from build123d import *

# Parameters (mm, degrees)
SKETCH_1_W          = 57
SKETCH_1_H          = 57
EXTRUDE_1_DEPTH     = 112
FILLET_1_R          = 2
CUT_EXTRUDE_2_DEPTH = 107.3
SKETCH_6_R          = 4
EXTRUDE_2_DEPTH     = 20
SKETCH_7_W          = 9.44271558
SKETCH_7_H          = 0.5
CUT_EXTRUDE_3_DEPTH = 15
SKETCH_2_R          = 19.05
EXTRUDE_3_DEPTH     = 1.5
SKETCH_8_R          = 2.6
CUT_EXTRUDE_4_DEPTH = 4.7


with BuildPart() as part:
    # 草图1 → 凸台-拉伸1 (new body)
    with BuildSketch(Plane(origin=(0, 0, 0), x_dir=(0, 0, -1), z_dir=(1, 0, 0))):
        Rectangle(SKETCH_1_W, SKETCH_1_H)
    extrude(amount=EXTRUDE_1_DEPTH)

    # 圆角1
    fillet_1_edges = [part.edges().sort_by_distance(p)[0] for p in [
        (56, 28.5, 28.5),
        (56, 28.5, -28.5),
        (56, -28.5, -28.5),
        (56, -28.5, 28.5),
    ]]
    fillet(fillet_1_edges, radius=FILLET_1_R)

    # 草图5 → 切除-拉伸2 (cut)
    with BuildSketch(Plane(origin=(112, 0, 0), x_dir=(0, 0, -1), z_dir=(1, 0, 0))):
        Polygon((-20.9, 20.9), (20.9, 20.9), (28.5, 20.9), (28.5, 28.5), (-28.5, 28.5), (-28.5, 20.9), align=None)
        Polygon((-28.5, -28.5), (28.5, -28.5), (28.5, -20.9), (20.9, -20.9), (-20.9, -20.9), (-28.5, -20.9), align=None)
    extrude(amount=-CUT_EXTRUDE_2_DEPTH, mode=Mode.SUBTRACT)

    # 草图6 → 凸台-拉伸2 (add)
    with BuildSketch(Plane.ZY):
        with Locations(Location((0, 0, 0), (0, 0, 180))):
            Circle(SKETCH_6_R)
    extrude(amount=EXTRUDE_2_DEPTH)

    # 草图7 → 切除-拉伸3 (cut)
    with BuildSketch(Plane.ZY.offset(20)):
        with Locations((0.062351887, 3.75)):
            Rectangle(SKETCH_7_W, SKETCH_7_H)
    extrude(amount=-CUT_EXTRUDE_3_DEPTH, mode=Mode.SUBTRACT)

    # 草图2 → 凸台-拉伸3 (add)
    with BuildSketch(Plane.ZY):
        with Locations(Location((0, 0, 0), (0, 0, 180))):
            Circle(SKETCH_2_R)
    extrude(amount=EXTRUDE_3_DEPTH)

    # 草图8 → 切除-拉伸4 (cut)
    with BuildSketch(Plane.ZY):
        with Locations((-23.5, 23.5)):
            Circle(SKETCH_8_R)
        with Locations((23.5, 23.5)):
            Circle(SKETCH_8_R)
        with Locations((-23.5, -23.5)):
            Circle(SKETCH_8_R)
        with Locations((23.5, -23.5)):
            Circle(SKETCH_8_R)
    extrude(amount=-CUT_EXTRUDE_4_DEPTH, mode=Mode.SUBTRACT)


solid = part.part
Work out the finished part from the listing and answer in its coordinate system (mm). A direction names the side the tool comes from. Give positions to 0.01 mm unless a question says otherwise; leave off trailing zeros. Order: outer loops, then holes, each group sorted by start corner. A loop starts at its lowest first (then second) coordinate and runs counter-clockwise, first axis right, second up. Notation, with made-up numbers: (-29, 67.5) -> (-3, 67.5) arc R24 cw to (-3, 98.5) -> close; hole circle Ø11 at (-2.75, 68). An arc over 180 degrees is marked (long way). Answer as a JSON object with one key per item and string values. Group by question number.
1. A tool of negligible diameter and unlimited length cuts with its end or side. For faces 4 (the flat face through (4.7, -25, 0)), 5 (the flat face through (-13, 3.5, 0)), 6 (the flat face through (59, 20.9, 0)), 7 (the cylindrical face through (-10.62, -3.966, 0.521)), from which of +Z, -Z, +X, -X, +Y, -Y can it reach the whole face along a straight path? Write none if from no direction.
2. Flat-ended cylindrical pins translate along their axes: pin 1 Ø4 at (y, z) = (-23.5, -23.5) entering from -X; pin 2 Ø19 at (y, z) = (3, -9) entering from -X; pin 3 Ø6 at (y, z) = (23.5, 23.5) entering from -X; pin 4 Ø5 at (x, z) = (16.5, -1) entering from -Y. Find the tip coordinate at first contact, or state that the pin passes through.
3. The mould has two halves that part along Z. Classify faces 1 (the flat face through (4.7, 25, 0)), 2 (the cylindrical face through (-0.74, 18.597, 4.13)), 3 (the cylindrical face through (2.32, -21.31, 24.9)): released by +Z, released by -Z, zero draft, split by the parting line, or undercut.
4. Section A-A on y = 23.5 is taken. Determine the outline of the cut face in (x, z).
5. Consider line 1 along Y through (x, z) = (1.55, 23.5); line 2 along Y through (x, z) = (12, 5.5). Determine where each line is inside the solid, lowest interval first. Write a range as [from, to].
6. Section D-D on x = 98.5 is taken. Determine the outline of the cut face in (y, z).
7. Section C-C on y = 0 is taken. Determine the outline of the cut face in (x, z), plus the area to 3 significant figures.
8. Section B-B on z = 0 is taken. Determine the outline of the cut face in (x, y), plus the area to 3 significant figures.
Result sheet:
{
 "1": {"face 4": "+Z, -Z, +X, -Y", "face 5": "+Z, -Z, -X, +Y", "face 6": "+Z, -Z, +X, +Y", "face 7": "-X"},
 "2": {"pin 1": "passes through", "pin 2": "stops at x = -20", "pin 3": "stops at x = 0", "pin 4": "stops at y = -20.9"},
 "3": {"face 1": "zero draft", "face 2": "split by the parting line", "face 3": "undercut"},
 "4": {"outline": "(0, -28.5) -> (4.7, -28.5) -> (4.7, -26.1) -> (0, -26.1) -> close; (0, -20.9) -> (4.7, -20.9) -> (4.7, 20.9) -> (0, 20.9) -> close; (0, 26.1) -> (4.7, 26.1) -> (4.7, 28.5) -> (0, 28.5) -> close"},
 "5": {"line 1": "y = [-28.5, -26.1], [-20.9, 20.9], [26.1, 28.5]", "line 2": "y = [-20.9, 20.9]"},
 "6": {"outline": "(-20.9, -28.5) -> (20.9, -28.5) -> (20.9, 28.5) -> (-20.9, 28.5) -> close"},
 "7": {"outline": "(-20, -4) -> (-1.5, -4) -> (-1.5, -19.05) -> (0, -19.05) -> (0, -28.5) -> (112, -28.5) -> (112, 28.5) -> (0, 28.5) -> (0, 19.05) -> (-1.5, 19.05) -> (-1.5, 4) -> (-20, 4) -> close", "area": "6,590 mm^2"},
 "8": {"outline": "(-20, -4) -> (-1.5, -4) -> (-1.5, -19.05) -> (0, -19.05) -> (0, -28.5) -> (4.7, -28.5) -> (4.7, -20.9) -> (112, -20.9) -> (112, 20.9) -> (4.7, 20.9) -> (4.7, 28.5) -> (0, 28.5) -> (0, 19.05) -> (-1.5, 19.05) -> (-1.5, 4) -> (-5, 4) -> (-5, 3.5) -> (-20, 3.5) -> close", "area": "4,950 mm^2"}
}
